Geometry check sheet. Reference: drawing and pictorial views, mm from the part's lowest x, y, z. A direction names the side the tool comes from. Give positions to 0.01 mm unless a question says otherwise; leave off trailing zeros. Order: outer loops, then holes, each group sorted by start corner. A loop starts at its lowest first (then second) coordinate and runs counter-clockwise, first axis right, second up.
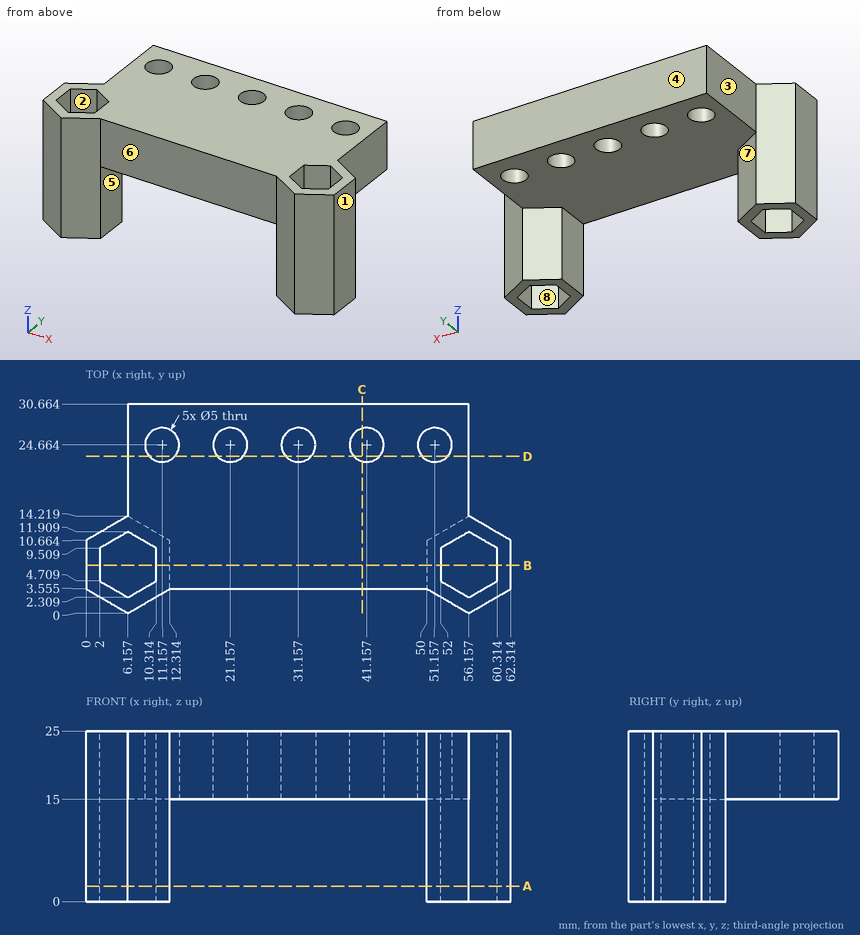
(1) Cross-section at B-B on y = 7. Enter the section's corners in (x, z).
Response values:
outline: (0, 0) - (2, 0) - (2, 25) - (0, 25) - close; (10.31, 0) - (12.31, 0) - (12.31, 15) - (50, 15) - (50, 0) - (52, 0) - (52, 25) - (10.31, 25) - close; (60.31, 0) - (62.31, 0) - (62.31, 25) - (60.31, 25) - close
(2) Cross-section at D-D on y = 23. Enter the section's corners in (x, z).
Response values:
outline: (6.16, 15) - (9.29, 15) - (9.29, 25) - (6.16, 25) - close; (13.02, 15) - (19.29, 15) - (19.29, 25) - (13.02, 25) - close; (23.02, 15) - (29.29, 15) - (29.29, 25) - (23.02, 25) - close; (33.02, 15) - (39.29, 15) - (39.29, 25) - (33.02, 25) - close; (43.02, 15) - (49.29, 15) - (49.29, 25) - (43.02, 25) - close; (53.02, 15) - (56.16, 15) - (56.16, 25) - (53.02, 25) - close
(3) Release check for a two-part mould opening along X. For the marked faces 1, 2, 3 and 4 record: released by +X, released by -X, zero draft, split by the parting line, or undercut.
Response values:
face 1: released by +X
face 2: undercut
face 3: released by -X
face 4: zero draft
(4) Cross-section at C-C on x = 40.5. Enter the section's corners in (y, z) (1 decimal).
Response values:
outline: (3.6, 15) - (22.3, 15) - (22.3, 25) - (3.6, 25) - close; (27.1, 15) - (30.7, 15) - (30.7, 25) - (27.1, 25) - close
(5) Set-up check for the marked faces 5, 6, 7 and 8: record each of +Z, -Z, +X, -X, +Y, -Y from which the full face is reachable in a straight line by a thin tool's end or side.
Response values:
face 5: -Z, +Y, -Y
face 6: +Z, -Z, -Y
face 7: -Z, +Y
face 8: +Z, -Z
(6) Cross-section at A-A on z = 2.25. Enter the section's corners in (x, y) (1 decimal).
Response values:
outline: (0, 3.6) - (6.2, 0) - (12.3, 3.6) - (12.3, 10.7) - (6.2, 14.2) - (0, 10.7) - close; (50, 3.6) - (56.2, 0) - (62.3, 3.6) - (62.3, 10.7) - (56.2, 14.2) - (50, 10.7) - close; hole (2, 4.7) - (6.2, 2.3) - (10.3, 4.7) - (10.3, 9.5) - (6.2, 11.9) - (2, 9.5) - close; hole (52, 4.7) - (56.2, 2.3) - (60.3, 4.7) - (60.3, 9.5) - (56.2, 11.9) - (52, 9.5) - close
(7) Material ranges on L1, parallel to X at y = 6.5, z = 21.75; L2, parallel to X at y = 6.5, z = 5.5; L3, parallel to Z at x = 48, y = 24.5, recorded low to high.
Response values:
L1: x = 0 to 2, 10.31 to 52, 60.31 to 62.31
L2: x = 0 to 2, 10.31 to 12.31, 50 to 52, 60.31 to 62.31
L3: z = 15 to 25
(8) Gauge pin test, flat ends, axial feed: pin 1 Ø12 at (y, z) = (14, 12.5) entering from +X; pin 2 Ø6.5 at (x, y) = (51.16, 24.66) entering from -Z; pin 3 Ø5 at (y, z) = (23, 21.5) entering from -X; pin 4 Ø3 at (y, z) = (19.5, 19) entering from +X. Record the tip position at first contact, or that the pin passes through.
Response values:
pin 1: stops at x = 62.31
pin 2: stops at z = 15
pin 3: stops at x = 6.16
pin 4: stops at x = 56.16
